from build123d import *

# Parameters (mm, degrees)
BOSS_EXTRU_1_DEPTH = 250
ESQUISSE7_W        = 3
ESQUISSE7_H        = 250
BOSS_EXTRU_4_DEPTH = 60


with BuildPart() as part:
    # Esquisse1 → Boss.-Extru.1 (new body)
    with BuildSketch(Plane(origin=(0, 0, 0), x_dir=(1, 0, 0), z_dir=(0, 1, 0))):
        with BuildLine():
            ThreePointArc((74, 0), (65.667169842, 34.11484728), (42.545329596, 60.546634337))
            Line((42.545329596, 60.546634337), (40.820518937, 58.092041053))
            ThreePointArc((40.820518937, 58.092041053), (63.004987281, 32.731812931), (71, 0))
            ThreePointArc((71, 0), (32.731812931, -63.004987281), (-40.820518937, -58.092041053))
            Line((-40.820518937, -58.092041053), (-42.545329596, -60.546634337))
            ThreePointArc((-42.545329596, -60.546634337), (34.11484728, -65.667169842), (74, 0))
        make_face()
    extrude(amount=BOSS_EXTRU_1_DEPTH)

    # Esquisse7 → Boss.-Extru.4 (add)
    with BuildSketch(Plane(origin=(0, 0, 0), x_dir=(-0.5749368864324517, 0, 0.8181977613140713), z_dir=(-0.8181977613140715, 0, -0.5749368864324517))):
        with Locations((-72.5, 125)):
            Rectangle(ESQUISSE7_W, ESQUISSE7_H)
    extrude(amount=BOSS_EXTRU_4_DEPTH)


solid = part.part
Design review of the part built by this model. Coordinates are the model's own, in mm. Coordinates: 2 decimals unless noted, no trailing zeros. Loops run counter-clockwise (first coordinate to the right, second up) from the corner with the lowest first, then second, coordinate; pieces in that order, holes last. Notation, with made-up numbers: (27, 31) - (84, 31) arc R4 ccw to (84, 35) - close; hole circle Ø7 at (66, -29.75). An arc over 180 degrees is marked (long way). Use CSV: the item, a comma, the result in double quotes. Start each with the question number.
1. To check wall thickness, follow probe 1 along Z at (x, y) = (59, 145); probe 2 along Z at (x, y) = (10.5, 52); probe 3 along X at (y, z) = (197.5, 63.5). State the ranges of each line that lie inside material, in increasing order.
2. Add section A-A on x = -3.5. Give the boundary of the cut face in (y, z).
3. Clearance check with flat-ended pins moving along their axes: pin 1 (4 mm diameter, centred on x = 15, y = 119, fed in from -Z); pin 2 (5 mm diameter, centred on y = 119.5, z = -37, fed in from +X); pin 3 (6 mm diameter, centred on y = 217.5, z = 35.5, fed in from -X). State where each tip first meets the part, or that it passes through.
4. Add section C-C on x = 49. Give the boundary of the cut face in (y, z), plus the area to 3 significant figures.
5. Add section D-D on z = -13.5. Give the boundary of the cut face in (x, y), plus the area to 3 significant figures.
6. Mouldability with a two-part tool opening along Z and no side actions: class faces 1 (the flat face through (18.343, 123.25, -77.553)), 2 (the flat face through (71, 250, -11)), 3 (the flat face through (16.618, 123.25, -75.099)) as released by +Z, released by -Z, zero draft, split by the parting line, or undercut.
Resolved:
1,probe 1,"-44.67 to -39.5, 39.5 to 44.67"
1,probe 2,"-83.06 to -79.4, 70.22 to 73.25"
1,probe 3,"-38 to -31.76, 31.76 to 38"
2,outline,"(0, -92.9) - (250, -92.9) - (250, -89.24) - (0, -89.24) - close; (0, 70.91) - (250, 70.91) - (250, 73.92) - (0, 73.92) - close"
3,pin 1,"z = -81.31"
3,pin 2,"x = 65.47"
3,pin 3,"x = 59.66"
4,outline,"(0, -55.45) - (250, -55.45) - (250, -51.38) - (0, -51.38) - close; (0, 51.38) - (250, 51.38) - (250, 55.45) - (0, 55.45) - close"
4,area,"2,040 mm2"
5,outline,"(69.7, 0) - (72.76, 0) - (72.76, 250) - (69.7, 250) - close"
5,area,"763 mm2"
6,face 1,"released by -Z"
6,face 2,"zero draft"
6,face 3,"undercut"
